Read the model definition and answer for the solid it produces. Units are mm, in the model's axes. Face numbers are marked on the shaded views. Coordinates: 2 decimals unless noted, no trailing zeros. Write each loop counter-clockwise with the first axis right and the second up, starting at its lowest first coordinate (ties: lowest second). Pieces come first, ordered by that corner, then holes.
(1) Section B-B on z = 22.5 is taken. Write down the section's boundary in (x, y), then the cut area to 3 significant figures.
(2) Section C-C on x = -22.5 is taken. Write down the section's boundary in (y, z), then the cut area to 3 significant figures.
(3) The mould has two halves that part along Z. Classify the marked faces 1, 2 and 3: +Z half, -Z half, draft (parallel to the pull), parting line (faces both ways), or undercut.
(4) Given pin 1 (6 mm diameter, centred on y = -8.5, z = 16.5, fed in from -X); pin 2 (1.5 mm diameter, centred on y = 35.5, z = 12.5, fed in from -X); pin 3 (3 mm diameter, centred on x = -4, z = 17, fed in from +Y); pin 4 (4 mm diameter, centred on x = -22, y = 9, fed in from +Z), each flat-ended and moving along its own axis, determine where each tip first touches the part or whether it passes through.
(5) Find the intervals of material crossed by probe 1 along Z at (x, y) = (-21, 40); probe 2 along Z at (x, y) = (-6, 12.5); probe 3 along X at (y, z) = (40, 4), in increasing order.
(6) Section A-A on y = 23.5 is taken. Write down the section's boundary in (x, z).
from build123d import *

# Parameters (mm, degrees)
F1_W     = 23.8884352148
F1_H     = 65.4788929969
F3_DEPTH = 9.144


with BuildPart() as f2:
    # F2: sweep along a path in F0
    with BuildLine(Plane.XZ) as f2_path:
        ThreePointArc((0, 0), (-5.1494897323, 17.4114904643), (-19.9215319008, 27.9691424221))
    # F1 (on Top) → F2 (sweep)
    with BuildSketch(Plane.XY):
        with Locations((-11.9442176074, 16.281622462)):
            Rectangle(F1_W, F1_H)
    sweep(path=f2_path.line)

    # F3 (add): a face of the model
    f3_faces = [f2.faces().sort_by_distance(p)[0] for p in [
        (-22.82294692, 16.281622462, 16.3826794096),
    ]]
    extrude(f3_faces, amount=F3_DEPTH)


solid = f2.part
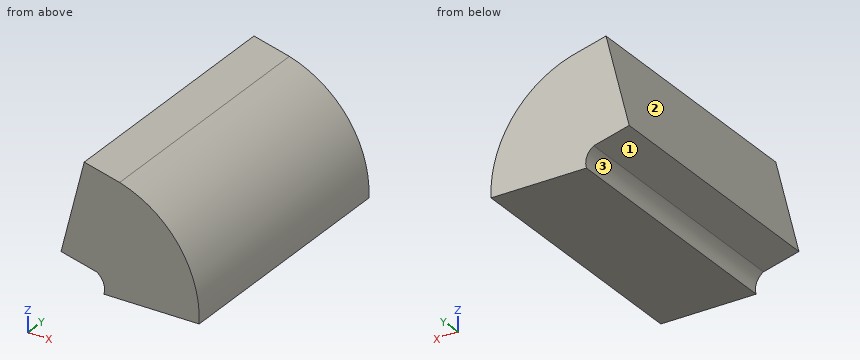
Response:
1. outline: (-30.72, -16.46) - (-9.82, -16.46) - (-9.82, 49.02) - (-30.72, 49.02) - close
1. area: 1,370 mm2
2. outline: (-16.46, 0) - (49.02, 0) - (49.02, 28.61) - (-16.46, 28.61) - close
2. area: 1,870 mm2
3. face 1: -Z half
3. face 2: +Z half
3. face 3: undercut
4. pin 1: stops at x = -32.97
4. pin 2: stops at x = -33.41
4. pin 3: stops at y = 49.02
4. pin 4: stops at z = 28.99
5. probe 1: z = 0 to 28.24
5. probe 2: z = 0 to 18.54
5. probe 3: x = -24.76 to -0.11
6. outline: (-34.59, 7.02) - (-25.72, 4.8) arc R4.17 cw to (-23.89, 0) - (0, 0) arc R27.91 ccw to (-19.92, 27.97) - (-28.79, 30.19) - close
